Work out the finished part from the listing and answer in its coordinate system (mm). Face numbers are marked on the shaded views. A direction names the side the tool comes from. Round coordinates to 2 decimals unless told otherwise and drop trailing zeros. Loops run counter-clockwise (first coordinate to the right, second up) from the corner with the lowest first, then second, coordinate; pieces in that order, holes last. Notation, with made-up numbers: (-28, 43) - (0, 43) arc R34 cw to (0, 82) - close; hole circle Ø1 at (-30.5, 6.25). An arc over 180 degrees is marked (long way). Return JSON: item names as keys, results as strings.
from build123d import *
from build123d.topology import SkipClean

# Parameters (mm, degrees)
SKETCH_1_W           = 42.7
SKETCH_1_H           = 21
SKETCH_1_R           = 1.5
EXTRUDE_1_DEPTH      = 2
SKETCH_2_R           = 1.25
SKETCH_2_R_2         = 3
EXTRUDE_2_DEPTH      = 2
EXTRUDE_3_DEPTH      = 1
EXTRUDE_3_DEPTH_BACK = 3
SKETCH_3_W           = 42.7
SKETCH_3_H           = 21
SKETCH_4_R           = 10.5
SKETCH_4_R_2         = 1.5
EXTRUDE_4_DEPTH      = 3
FILLET_1_R           = 10
FILLET_2_R           = 5
CUT_EXTRUDE_START    = -4
SKETCH_6_R           = 1.5
CUT_EXTRUDE_1_DEPTH  = 4


with BuildPart() as part:
    # 草图1 → 凸台-拉伸1 (new body)
    with BuildSketch(Plane(origin=(0, 0, 0), x_dir=(1, 0, 0), z_dir=(0, 1, 0))):
        Rectangle(SKETCH_1_W, SKETCH_1_H)
        with Locations(Location((7.5, 5, 0), (0, 0, 270))):
            Circle(SKETCH_1_R, mode=Mode.SUBTRACT)
        with Locations(Location((7.5, -5, 0), (0, 0, 90))):
            Circle(SKETCH_1_R, mode=Mode.SUBTRACT)
        with Locations(Location((-7.5, -5, 0), (0, 0, 270))):
            Circle(SKETCH_1_R, mode=Mode.SUBTRACT)
        with Locations(Location((-7.5, 5, 0), (0, 0, 90))):
            Circle(SKETCH_1_R, mode=Mode.SUBTRACT)
        with BuildLine():
            Line((8.017950723, 1.550908082), (12.912587519, 1.550908082))
            ThreePointArc((12.912587519, 1.550908082), (14.126270768, 1.145131224), (14.697546856, 0))
            ThreePointArc((14.697546856, 0), (14.126270768, -1.145131224), (12.912587519, -1.550908082))
            Line((12.912587519, -1.550908082), (8.017950723, -1.550908082))
            add(Edge.make_bspline(
                [(0, -7.407271614), (2.092471107, -7.358009404), (3.043739342, -2.951912586), (6.007732496, -1.626733157), (8.017950723, -1.550908082)],
                knots=[0, 0, 0, 0, 0.496822763, 1, 1, 1, 1], degree=3))
            add(Edge.make_bspline(
                [(0, -7.407271614), (-2.092471107, -7.358009404), (-3.043739342, -2.951912586), (-6.007732496, -1.626733157), (-8.017950723, -1.550908082)],
                knots=[0, 0, 0, 0, 0.496822763, 1, 1, 1, 1], degree=3))
            Line((-8.017950723, -1.550908082), (-12.912587519, -1.550908082))
            ThreePointArc((-12.912587519, -1.550908082), (-14.126270768, -1.145131224), (-14.697546856, 0))
            ThreePointArc((-14.697546856, 0), (-14.126270768, 1.145131224), (-12.912587519, 1.550908082))
            Line((-12.912587519, 1.550908082), (-8.017950723, 1.550908082))
            add(Edge.make_bspline(
                [(0, 7.407271614), (-2.092471107, 7.358009404), (-3.043739342, 2.951912586), (-6.007732496, 1.626733157), (-8.017950723, 1.550908082)],
                knots=[0, 0, 0, 0, 0.496822763, 1, 1, 1, 1], degree=3))
            add(Edge.make_bspline(
                [(0, 7.407271614), (2.092471107, 7.358009404), (3.043739342, 2.951912586), (6.007732496, 1.626733157), (8.017950723, 1.550908082)],
                knots=[0, 0, 0, 0, 0.496822763, 1, 1, 1, 1], degree=3))
        make_face(mode=Mode.SUBTRACT)
    extrude(amount=EXTRUDE_1_DEPTH)

    # 草图2 → 凸台-拉伸2 (add)
    with BuildSketch(Plane.ZY.offset(21.35)):
        with BuildLine():
            Line((-10.5, 2), (-10.5, 46))
            ThreePointArc((-10.5, 46), (0, 56.5), (10.5, 46))
            Line((10.5, 46), (10.5, 2))
            Line((10.5, 2), (-10.5, 2))
        make_face()
        with Locations((0, 38.65)):
            Circle(SKETCH_2_R, mode=Mode.SUBTRACT)
        with Locations((-7.35, 46)):
            Circle(SKETCH_2_R, mode=Mode.SUBTRACT)
        with Locations((0, 53.35)):
            Circle(SKETCH_2_R, mode=Mode.SUBTRACT)
        with Locations((7.35, 46)):
            Circle(SKETCH_2_R, mode=Mode.SUBTRACT)
        with Locations((0, 46)):
            Circle(SKETCH_2_R_2, mode=Mode.SUBTRACT)
        with BuildLine():
            Line((-2.091438456, 33.71946821), (-2.091438456, 8.682620376))
            ThreePointArc((-2.091438456, 8.682620376), (-4.622608783, 10.734209017), (-5.574745456, 13.850179963))
            Line((-5.574745456, 13.850179963), (-5.574745456, 28.551908623))
            ThreePointArc((-5.574745456, 28.551908623), (-4.622608783, 31.667879569), (-2.091438456, 33.71946821))
        make_face(mode=Mode.SUBTRACT)
        with BuildLine():
            Line((5.574745456, 28.551908623), (5.574745456, 13.850179963))
            ThreePointArc((5.574745456, 13.850179963), (4.622608783, 10.734209017), (2.091438456, 8.682620376))
            Line((2.091438456, 8.682620376), (2.091438456, 33.71946821))
            ThreePointArc((2.091438456, 33.71946821), (4.622608783, 31.667879569), (5.574745456, 28.551908623))
        make_face(mode=Mode.SUBTRACT)
    extrude_2 = extrude(amount=-EXTRUDE_2_DEPTH)

    # 镜向1: 凸台-拉伸2 across plane
    add(extrude_2.mirror(Plane(origin=(0, 0, 0), x_dir=(0, 0, 1), z_dir=(1, 0, 0))))

    # 草图3 → 凸台-拉伸3 (add, two sides: drawn at the far end of the back side and taken through both)
    with BuildSketch(Plane.XZ.offset(-EXTRUDE_3_DEPTH_BACK)):
        Rectangle(SKETCH_3_W, SKETCH_3_H)
    extrude(amount=EXTRUDE_3_DEPTH + EXTRUDE_3_DEPTH_BACK)

    # 草图4 → 凸台-拉伸4 (add)
    with BuildSketch(Plane.XZ.offset(1)):
        with Locations(Location((0, 0, 0), (0, 0, 270))):
            Circle(SKETCH_4_R)
        with Locations(Location((0, 7, 0), (0, 0, 270))):
            Circle(SKETCH_4_R_2, mode=Mode.SUBTRACT)
        with Locations(Location((0, -7, 0), (0, 0, 270))):
            Circle(SKETCH_4_R_2, mode=Mode.SUBTRACT)
    extrude(amount=EXTRUDE_4_DEPTH)

    # 圆角1
    # the kernel refuses this fillet: 10 mm, written as the material it adds along each edge
    with BuildSketch(Plane(origin=(19.35, 3, -10.5), x_dir=(-1, 0, 0), z_dir=(0, 0, 1))) as fillet_1_piece_1_section:
        with BuildLine():
            CenterArc((FILLET_1_R, -FILLET_1_R), FILLET_1_R, 90, 90)
            Line((0, -FILLET_1_R), (0, 0))
            Line((0, 0), (FILLET_1_R, 0))
        make_face()
    fillet_1_piece_1 = extrude(amount=21, mode=Mode.PRIVATE)
    fillet_1_piece_1 = fillet_1_piece_1 - Plane(origin=(17.043313865, 13.850179963, 0), x_dir=(0, 0, 1), z_dir=(1, 0, 0)) * Cylinder(5.574745456, 82, mode=Mode.PRIVATE)
    fillet_1_piece_1 = split(fillet_1_piece_1, bisect_by=Plane(origin=(17.043313865, 5.15733044, -2.091438456), z_dir=(0, 0, -1)), keep=Keep.TOP, mode=Mode.PRIVATE)
    add(fillet_1_piece_1)
    with BuildSketch(Plane(origin=(19.35, 3, -10.5), x_dir=(-1, 0, 0), z_dir=(0, 0, 1))) as fillet_1_piece_2_section:
        with BuildLine():
            CenterArc((FILLET_1_R, -FILLET_1_R), FILLET_1_R, 90, 90)
            Line((0, -FILLET_1_R), (0, 0))
            Line((0, 0), (FILLET_1_R, 0))
        make_face()
    fillet_1_piece_2 = extrude(amount=21, mode=Mode.PRIVATE)
    fillet_1_piece_2 = split(fillet_1_piece_2, bisect_by=Plane(origin=(16.850424397, 4.734237848, 2.091438456), z_dir=(0, 0, -1)), keep=Keep.TOP, mode=Mode.PRIVATE)
    fillet_1_piece_2 = fillet_1_piece_2 - Plane(origin=(16.850424397, 13.850179963, 0), x_dir=(0, 0, 1), z_dir=(1, 0, 0)) * Cylinder(5.574745456, 82, mode=Mode.PRIVATE)
    fillet_1_piece_2 = split(fillet_1_piece_2, bisect_by=Plane(origin=(16.850424397, 4.734237848, -2.091438456), z_dir=(0, 0, 1)), keep=Keep.TOP, mode=Mode.PRIVATE)
    add(fillet_1_piece_2)
    with BuildSketch(Plane(origin=(19.35, 3, -10.5), x_dir=(-1, 0, 0), z_dir=(0, 0, 1))) as fillet_1_piece_3_section:
        with BuildLine():
            CenterArc((FILLET_1_R, -FILLET_1_R), FILLET_1_R, 90, 90)
            Line((0, -FILLET_1_R), (0, 0))
            Line((0, 0), (FILLET_1_R, 0))
        make_face()
    fillet_1_piece_3 = extrude(amount=21, mode=Mode.PRIVATE)
    fillet_1_piece_3 = split(fillet_1_piece_3, bisect_by=Plane(origin=(19.170455524, 9.949953682, 2.091438456), z_dir=(0, 0, -1)), keep=Keep.TOP, mode=Mode.PRIVATE)
    fillet_1_piece_3 = fillet_1_piece_3 & Plane(origin=(19.170455524, 13.850179963, 0), x_dir=(0, 0, 1), z_dir=(1, 0, 0)) * Cylinder(5.574745456, 82, mode=Mode.PRIVATE)
    fillet_1_piece_3 = split(fillet_1_piece_3, bisect_by=Plane(origin=(19.170455524, 9.949953682, -2.091438456), z_dir=(0, 0, 1)), keep=Keep.TOP, mode=Mode.PRIVATE)
    add(fillet_1_piece_3)
    with BuildSketch(Plane(origin=(19.35, 3, -10.5), x_dir=(-1, 0, 0), z_dir=(0, 0, 1))) as fillet_1_piece_4_section:
        with BuildLine():
            CenterArc((FILLET_1_R, -FILLET_1_R), FILLET_1_R, 90, 90)
            Line((0, -FILLET_1_R), (0, 0))
            Line((0, 0), (FILLET_1_R, 0))
        make_face()
    fillet_1_piece_4 = extrude(amount=21, mode=Mode.PRIVATE)
    fillet_1_piece_4 = split(fillet_1_piece_4, bisect_by=Plane(origin=(17.043313289, 5.157330644, 2.091438456), z_dir=(0, 0, 1)), keep=Keep.TOP, mode=Mode.PRIVATE)
    fillet_1_piece_4 = fillet_1_piece_4 - Plane(origin=(17.043313289, 13.850179963, 0), x_dir=(0, 0, 1), z_dir=(1, 0, 0)) * Cylinder(5.574745456, 82, mode=Mode.PRIVATE)
    add(fillet_1_piece_4)
    with BuildSketch(Plane(origin=(-19.35, 3, -10.5), x_dir=(0, 1, 0), z_dir=(0, 0, 1))) as fillet_1_piece_5_section:
        with BuildLine():
            CenterArc((FILLET_1_R, -FILLET_1_R), FILLET_1_R, 90, 90)
            Line((0, -FILLET_1_R), (0, 0))
            Line((0, 0), (FILLET_1_R, 0))
        make_face()
    fillet_1_piece_5 = extrude(amount=21, mode=Mode.PRIVATE)
    fillet_1_piece_5 = fillet_1_piece_5 - Plane(origin=(-17.043313718, 13.850179963, 0), x_dir=(0, 0, 1), z_dir=(-1, 0, 0)) * Cylinder(5.574745456, 82, mode=Mode.PRIVATE)
    fillet_1_piece_5 = split(fillet_1_piece_5, bisect_by=Plane(origin=(-17.043313718, 5.157330569, -2.091438456), z_dir=(0, 0, -1)), keep=Keep.TOP, mode=Mode.PRIVATE)
    add(fillet_1_piece_5)
    with BuildSketch(Plane(origin=(-19.35, 3, -10.5), x_dir=(0, 1, 0), z_dir=(0, 0, 1))) as fillet_1_piece_6_section:
        with BuildLine():
            CenterArc((FILLET_1_R, -FILLET_1_R), FILLET_1_R, 90, 90)
            Line((0, -FILLET_1_R), (0, 0))
            Line((0, 0), (FILLET_1_R, 0))
        make_face()
    fillet_1_piece_6 = extrude(amount=21, mode=Mode.PRIVATE)
    fillet_1_piece_6 = split(fillet_1_piece_6, bisect_by=Plane(origin=(-16.850424159, 4.734237852, 2.091438456), z_dir=(0, 0, -1)), keep=Keep.TOP, mode=Mode.PRIVATE)
    fillet_1_piece_6 = fillet_1_piece_6 - Plane(origin=(-16.850424159, 13.850179963, 0), x_dir=(0, 0, 1), z_dir=(-1, 0, 0)) * Cylinder(5.574745456, 82, mode=Mode.PRIVATE)
    fillet_1_piece_6 = split(fillet_1_piece_6, bisect_by=Plane(origin=(-16.850424159, 4.734237852, -2.091438456), z_dir=(0, 0, 1)), keep=Keep.TOP, mode=Mode.PRIVATE)
    add(fillet_1_piece_6)
    with BuildSketch(Plane(origin=(-19.35, 3, -10.5), x_dir=(0, 1, 0), z_dir=(0, 0, 1))) as fillet_1_piece_7_section:
        with BuildLine():
            CenterArc((FILLET_1_R, -FILLET_1_R), FILLET_1_R, 90, 90)
            Line((0, -FILLET_1_R), (0, 0))
            Line((0, 0), (FILLET_1_R, 0))
        make_face()
    fillet_1_piece_7 = extrude(amount=21, mode=Mode.PRIVATE)
    fillet_1_piece_7 = split(fillet_1_piece_7, bisect_by=Plane(origin=(-17.043313652, 5.157330325, 2.091438456), z_dir=(0, 0, 1)), keep=Keep.TOP, mode=Mode.PRIVATE)
    fillet_1_piece_7 = fillet_1_piece_7 - Plane(origin=(-17.043313652, 13.850179963, 0), x_dir=(0, 0, 1), z_dir=(-1, 0, 0)) * Cylinder(5.574745456, 82, mode=Mode.PRIVATE)
    add(fillet_1_piece_7)
    with BuildSketch(Plane(origin=(-19.35, 3, -10.5), x_dir=(0, 1, 0), z_dir=(0, 0, 1))) as fillet_1_piece_8_section:
        with BuildLine():
            CenterArc((FILLET_1_R, -FILLET_1_R), FILLET_1_R, 90, 90)
            Line((0, -FILLET_1_R), (0, 0))
            Line((0, 0), (FILLET_1_R, 0))
        make_face()
    fillet_1_piece_8 = extrude(amount=21, mode=Mode.PRIVATE)
    fillet_1_piece_8 = split(fillet_1_piece_8, bisect_by=Plane(origin=(-19.170455532, 9.949953694, 2.091438456), z_dir=(0, 0, -1)), keep=Keep.TOP, mode=Mode.PRIVATE)
    fillet_1_piece_8 = fillet_1_piece_8 & Plane(origin=(-19.170455532, 13.850179963, 0), x_dir=(0, 0, 1), z_dir=(-1, 0, 0)) * Cylinder(5.574745456, 82, mode=Mode.PRIVATE)
    fillet_1_piece_8 = split(fillet_1_piece_8, bisect_by=Plane(origin=(-19.170455532, 9.949953694, -2.091438456), z_dir=(0, 0, 1)), keep=Keep.TOP, mode=Mode.PRIVATE)
    add(fillet_1_piece_8)

    # 圆角2
    fillet_2_edges = [part.edges().sort_by_distance(p)[0] for p in [
        (-21.35, -1, 0),
        (21.35, -1, 0),
    ]]
    fillet(fillet_2_edges, radius=FILLET_2_R)

    # 草图6 → 切除-拉伸1 (cut)
    with SkipClean():  # the faces are left unmerged after this step: merging them gives an invalid solid
        with BuildSketch(Plane.XZ.offset(1).offset(CUT_EXTRUDE_START)):
            with Locations(Location((0, 7, 0), (0, 0, 270))):
                Circle(SKETCH_6_R)
            with Locations(Location((0, -7, 0), (0, 0, 270))):
                Circle(SKETCH_6_R)
        extrude(amount=CUT_EXTRUDE_1_DEPTH, mode=Mode.SUBTRACT)


solid = part.part
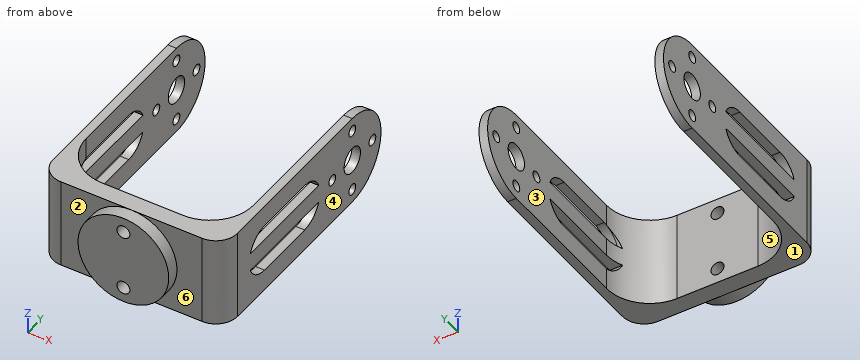
1) Flat-ended cylindrical pins translate along their axes: pin 1 (3 mm diameter, centred on y = 46, z = 7.35, fed in from +X); pin 2 (5 mm diameter, centred on x = 0, z = 7, fed in from +Y); pin 3 (5 mm diameter, centred on x = 15, z = -6.5, fed in from -Y); pin 4 (2 mm diameter, centred on y = 38.65, z = 0, fed in from -X). Find the tip coordinate at first contact, or state that the pin passes through.
Verdict:
{"pin 1": "stops at x = 21.35", "pin 2": "stops at y = 3", "pin 3": "stops at y = -1", "pin 4": "passes through"}
2) Section C-C (y = 38.65) is taken. Give the vertices of the cut face in (x, z), and give its area (3 significant figures).
Verdict:
{"outline": "(-21.35, -10.5) - (-19.35, -10.5) - (-19.35, -1.25) - (-21.35, -1.25) - close; (-21.35, 1.25) - (-19.35, 1.25) - (-19.35, 10.5) - (-21.35, 10.5) - close; (19.35, -10.5) - (21.35, -10.5) - (21.35, -1.25) - (19.35, -1.25) - close; (19.35, 1.25) - (21.35, 1.25) - (21.35, 10.5) - (19.35, 10.5) - close", "area": "74.0 mm2"}
3) Determine the mould class of the marked faces 4, 5 and 6 for opening direction X: pulls with the +X half, pulls with the -X half, needs draft (parallel to the pull), parting line crosses it, or undercut.
Verdict:
{"face 4": "pulls with the +X half", "face 5": "undercut", "face 6": "needs draft"}
4) A tool of negligible diameter and unlimited length cuts with its end or side. For the marked faces 1, 2 and 3, from which of +Z, -Z, +X, -X, +Y, -Y can it reach the whole face along a straight path? Write none if from no direction.
Verdict:
{"face 1": "-Z, +X, -X, +Y, -Y", "face 2": "-X, -Y", "face 3": "+Z, -Z, +Y"}
5) Find the intervals of material crossed by L1, parallel to Z at x = 19.5, y = 28; L2, parallel to X at y = 48, z = -2.75; L3, parallel to Y at x = -20.1, z = 0, in increasing order.
Verdict:
{"L1": "z = -10.5 to -5.57, -2.09 to 2.09, 5.57 to 10.5", "L2": "x = -21.35 to -19.35, 19.35 to 21.35", "L3": "y = 0.69 to 37.4, 39.9 to 43, 49 to 52.1, 54.6 to 56.5"}
6) Section B-B (z = 7.35) is taken. Give the vertices of the cut face in (x, y).
Verdict:
{"outline": "(-21.35, 4) arc R5 ccw to (-16.35, -1) - (-7.5, -1) - (-7.5, -4) - (-1.46, -4) - (-1.46, 3) - (-9.35, 3) arc R10 cw to (-19.35, 13) - (-19.35, 44.75) - (-21.35, 44.75) - close; (-21.35, 47.25) - (-19.35, 47.25) - (-19.35, 53.5) - (-21.35, 53.5) - close; (1.46, -4) - (7.5, -4) - (7.5, -1) - (16.35, -1) arc R5 ccw to (21.35, 4) - (21.35, 44.75) - (19.35, 44.75) - (19.35, 13) arc R10 cw to (9.35, 3) - (1.46, 3) - close; (19.35, 47.25) - (21.35, 47.25) - (21.35, 53.5) - (19.35, 53.5) - close"}
7) Section A-A (y = 53.35) is taken. Give the vertices of the cut face in (x, z), and give its area (3 significant figures).
Verdict:
{"outline": "(-21.35, -7.5) - (-19.35, -7.5) - (-19.35, -1.25) - (-21.35, -1.25) - close; (-21.35, 1.25) - (-19.35, 1.25) - (-19.35, 7.5) - (-21.35, 7.5) - close; (19.35, -7.5) - (21.35, -7.5) - (21.35, -1.25) - (19.35, -1.25) - close; (19.35, 1.25) - (21.35, 1.25) - (21.35, 7.5) - (19.35, 7.5) - close", "area": "50.0 mm2"}
8) Section D-D (z = 0) is taken. Count the separate pieces of the cut face and the enclosed holes in it, and give its area (3 significant figures).
Verdict:
{"separate pieces": "7", "enclosed holes": "0", "area": "436 mm2"}
